from build123d import *

# Parameters (mm, degrees)
SKETCH1_W           = 180
SKETCH1_H           = 30
BOSS_EXTRUDE1_DEPTH = 3
FILLET1_R           = 5
CUT_EXTRUDE1_DEPTH  = 92.290744328


# Read off the part's stored shape, not the designer's step: CSK for M3 Flat Head Machine Screw1
with BuildPart() as part:
    # Sketch1 → Boss-Extrude1 (new body)
    with BuildSketch(Plane.XY):
        Rectangle(SKETCH1_W, SKETCH1_H)
    extrude(amount=BOSS_EXTRUDE1_DEPTH)

    # Fillet1
    fillet1_edges = [part.edges().sort_by_distance(p)[0] for p in [
        (90, -15, 1.5),
        (-90, -15, 1.5),
        (-90, 15, 1.5),
        (90, 15, 1.5),
    ]]
    fillet(fillet1_edges, radius=FILLET1_R)

    # CSK for M3 Flat Head Machine Screw1 outl → CSK for M3 Flat Head Machine Screw1 (revolve, cut)
    with BuildSketch(Plane.XZ.offset(10)):
        Polygon((0, 0), (1.8, 0), (1.8, 1.4), (3.4, 3), (0, 3), align=None)
    revolve(axis=Axis((0, -10, 0), (0, 0, 1)), mode=Mode.SUBTRACT)

    # CSK for M3 Flat Head Machine Screw1 2 ou → CSK for M3 Flat Head Machine Screw1 2 (revolve, cut)
    with BuildSketch(Plane.XZ.offset(-10)):
        Polygon((0, 0), (1.8, 0), (1.8, 1.4), (3.4, 3), (0, 3), align=None)
    revolve(axis=Axis((0, 10, 0), (0, 0, 1)), mode=Mode.SUBTRACT)

    # CSK for M3 Flat Head Machine Screw1 3 ou → CSK for M3 Flat Head Machine Screw1 3 (revolve, cut)
    with BuildSketch(Plane(origin=(-84.5, -10, 0), x_dir=(1, 0, 0), z_dir=(0, -1, 0))):
        Polygon((0, 0), (1.8, 0), (1.8, 1.4), (3.4, 3), (0, 3), align=None)
    revolve(axis=Axis((-84.5, -10, 0), (0, 0, 1)), mode=Mode.SUBTRACT)

    # CSK for M3 Flat Head Machine Screw1 4 ou → CSK for M3 Flat Head Machine Screw1 4 (revolve, cut)
    with BuildSketch(Plane(origin=(84.5, 10, 0), x_dir=(1, 0, 0), z_dir=(0, -1, 0))):
        Polygon((0, 0), (1.8, 0), (1.8, 1.4), (3.4, 3), (0, 3), align=None)
    revolve(axis=Axis((84.5, 10, 0), (0, 0, 1)), mode=Mode.SUBTRACT)

    # CSK for M3 Flat Head Machine Screw1 5 ou → CSK for M3 Flat Head Machine Screw1 5 (revolve, cut)
    with BuildSketch(Plane(origin=(84.5, -10, 0), x_dir=(1, 0, 0), z_dir=(0, -1, 0))):
        Polygon((0, 0), (1.8, 0), (1.8, 1.4), (3.4, 3), (0, 3), align=None)
    revolve(axis=Axis((84.5, -10, 0), (0, 0, 1)), mode=Mode.SUBTRACT)

    # CSK for M3 Flat Head Machine Screw1 6 ou → CSK for M3 Flat Head Machine Screw1 6 (revolve, cut)
    with BuildSketch(Plane(origin=(-84.5, 10, 0), x_dir=(1, 0, 0), z_dir=(0, -1, 0))):
        Polygon((0, 0), (1.8, 0), (1.8, 1.4), (3.4, 3), (0, 3), align=None)
    revolve(axis=Axis((-84.5, 10, 0), (0, 0, 1)), mode=Mode.SUBTRACT)

    # Sketch5 → Cut-Extrude1 (cut, through all)
    with BuildSketch(Plane.XY.offset(3)):
        with BuildLine():
            Line((-85, -15), (85, -15))
            ThreePointArc((85, -15), (88.535533906, -13.535533906), (90, -10))
            Line((90, -10), (90, 10))
            ThreePointArc((90, 10), (88.535533906, 13.535533906), (85, 15))
            Line((85, 15), (-85, 15))
            ThreePointArc((-85, 15), (-88.535533906, 13.535533906), (-90, 10))
            Line((-90, 10), (-90, -10))
            ThreePointArc((-90, -10), (-88.535533906, -13.535533906), (-85, -15))
        make_face()
        with BuildLine():
            Line((-85, -14.7), (85, -14.7))
            ThreePointArc((85, -14.7), (88.323401872, -13.323401872), (89.7, -10))
            Line((89.7, -10), (89.7, 10))
            ThreePointArc((89.7, 10), (88.323401872, 13.323401872), (85, 14.7))
            Line((85, 14.7), (-85, 14.7))
            ThreePointArc((-85, 14.7), (-88.323401872, 13.323401872), (-89.7, 10))
            Line((-89.7, 10), (-89.7, -10))
            ThreePointArc((-89.7, -10), (-88.323401872, -13.323401872), (-85, -14.7))
        make_face(mode=Mode.SUBTRACT)
    extrude(amount=-CUT_EXTRUDE1_DEPTH, mode=Mode.SUBTRACT)


solid = part.part
Here's how the part is built. I have some questions about the finished solid (model axes, mm). Give positions to 0.01 mm unless a question says otherwise; leave off trailing zeros. Loops run counter-clockwise (first coordinate to the right, second up) from the corner with the lowest first, then second, coordinate; pieces in that order, holes last. Notation, with made-up numbers: (-5.75, 0.5) -> (29.25, 0.5) arc R16 ccw to (29.25, 27.5) -> close; hole circle Ø8 at (86.5, 29.5). An arc over 180 degrees is marked (long way). Answer as a JSON object with one key per item and string values. Group by question number.
Item 1: Imagine slicing it at A-A on z = 2.3. Write out the boundary of the cut face in (x, y), then the cut area to 3 significant figures.
Item 2: I need wall thicknesses on L1, parallel to X at y = 8, z = 2.3; L2, parallel to Y at x = -84.5, z = 0.45; L3, parallel to X at y = -9.5, z = 1.6. Which ranges of each line are inside material? Lowest first, please.
Item 3: Imagine slicing it at B-B on x = 0. Write out the boundary of the cut face in (y, z), then the cut area to 3 significant figures.
Item 4: Thinking about a two-plate mould opening in Y: for faces 1 (the cylindrical face through (88.36, 13.287, 1.521)), 2 (the cylindrical face through (-0.39, -11.757, 0.71)), 3 (the cylindrical face through (-86.3, -9.92, 0.71)), 4 (the cylindrical face through (88.287, -13.36, 1.521)), which applies, pulls with the +Y half, pulls with the -Y half, needs draft (parallel to the pull), parting line crosses it, or undercut?
Item 5: Will this pin go through, and if not, where does the flat tip stop? pin 1 (4.5 mm diameter, centred on x = 84.5, y = 10, fed in from +Z).
Answer list:
{
 "1": {"outline": "(-89.7, -10) arc R4.7 ccw to (-85, -14.7) -> (85, -14.7) arc R4.7 ccw to (89.7, -10) -> (89.7, 10) arc R4.7 ccw to (85, 14.7) -> (-85, 14.7) arc R4.7 ccw to (-89.7, 10) -> close; hole circle Ø5.4 at (-84.5, -10); hole circle Ø5.4 at (-84.5, 10); hole circle Ø5.4 at (0, -10); hole circle Ø5.4 at (0, 10); hole circle Ø5.4 at (84.5, -10); hole circle Ø5.4 at (84.5, 10)", "area": "5,120 mm2"},
 "2": {"L1": "x = -89.7 to -86.31, -82.69 to -1.81, 1.81 to 82.69, 86.31 to 89.7", "L2": "y = -14.7 to -11.8, -8.2 to 8.2, 11.8 to 14.7", "L3": "x = -89.7 to -86.44, -82.56 to -1.94, 1.94 to 82.56, 86.44 to 89.7"},
 "3": {"outline": "(-14.7, 0) -> (-11.8, 0) -> (-11.8, 1.4) -> (-13.4, 3) -> (-14.7, 3) -> close; (-8.2, 0) -> (8.2, 0) -> (8.2, 1.4) -> (6.6, 3) -> (-6.6, 3) -> (-8.2, 1.4) -> close; (11.8, 0) -> (14.7, 0) -> (14.7, 3) -> (13.4, 3) -> (11.8, 1.4) -> close", "area": "61.5 mm2"},
 "4": {"face 1": "pulls with the +Y half", "face 2": "undercut", "face 3": "undercut", "face 4": "pulls with the -Y half"},
 "5": {"pin 1": "stops at z = 1.85"}
}
